```python
from build123d import *

# Parameters (mm, degrees)
SKETCH1_R           = 1.778
BOSS_EXTRUDE1_DEPTH = 6.35
SKETCH2_R           = 1.778
BOSS_EXTRUDE2_DEPTH = 6.35
SKETCH3_R           = 1.905
CUT_EXTRUDE1_DEPTH  = 103.859220114


with BuildPart() as part:
    # Sketch1 → Boss-Extrude1 (new body)
    with BuildSketch(Plane(origin=(0, 6.35, 0), x_dir=(1, 0, 0), z_dir=(0, 1, 0))):
        with BuildLine():
            Line((97.79, 4.7625), (-97.79, 4.7625))
            ThreePointArc((-97.79, 4.7625), (-102.5525, 0), (-97.79, -4.7625))
            Line((-97.79, -4.7625), (97.79, -4.7625))
            ThreePointArc((97.79, -4.7625), (102.5525, 0), (97.79, 4.7625))
        make_face()
        with Locations(Location((97.79, 0, 0), (0, 0, 90))):
            Circle(SKETCH1_R, mode=Mode.SUBTRACT)
        with Locations(Location((88.011, 0, 0), (0, 0, 90))):
            Circle(SKETCH1_R, mode=Mode.SUBTRACT)
        with Locations(Location((78.232, 0, 0), (0, 0, 90))):
            Circle(SKETCH1_R, mode=Mode.SUBTRACT)
        with Locations(Location((68.453, 0, 0), (0, 0, 90))):
            Circle(SKETCH1_R, mode=Mode.SUBTRACT)
        with Locations(Location((58.674, 0, 0), (0, 0, 90))):
            Circle(SKETCH1_R, mode=Mode.SUBTRACT)
        with Locations(Location((48.895, 0, 0), (0, 0, 90))):
            Circle(SKETCH1_R, mode=Mode.SUBTRACT)
        with Locations(Location((39.116, 0, 0), (0, 0, 90))):
            Circle(SKETCH1_R, mode=Mode.SUBTRACT)
        with Locations(Location((29.337, 0, 0), (0, 0, 90))):
            Circle(SKETCH1_R, mode=Mode.SUBTRACT)
        with Locations(Location((19.558, 0, 0), (0, 0, 90))):
            Circle(SKETCH1_R, mode=Mode.SUBTRACT)
        with Locations(Location((9.779, 0, 0), (0, 0, 90))):
            Circle(SKETCH1_R, mode=Mode.SUBTRACT)
        with Locations(Location((0, 0, 0), (0, 0, 90))):
            Circle(SKETCH1_R, mode=Mode.SUBTRACT)
        with Locations(Location((-9.779, 0, 0), (0, 0, 90))):
            Circle(SKETCH1_R, mode=Mode.SUBTRACT)
        with Locations(Location((-19.558, 0, 0), (0, 0, 90))):
            Circle(SKETCH1_R, mode=Mode.SUBTRACT)
        with Locations(Location((-29.337, 0, 0), (0, 0, 90))):
            Circle(SKETCH1_R, mode=Mode.SUBTRACT)
        with Locations(Location((-39.116, 0, 0), (0, 0, 90))):
            Circle(SKETCH1_R, mode=Mode.SUBTRACT)
        with Locations(Location((-48.895, 0, 0), (0, 0, 90))):
            Circle(SKETCH1_R, mode=Mode.SUBTRACT)
        with Locations(Location((-58.674, 0, 0), (0, 0, 90))):
            Circle(SKETCH1_R, mode=Mode.SUBTRACT)
        with Locations(Location((-68.453, 0, 0), (0, 0, 90))):
            Circle(SKETCH1_R, mode=Mode.SUBTRACT)
        with Locations(Location((-78.232, 0, 0), (0, 0, 90))):
            Circle(SKETCH1_R, mode=Mode.SUBTRACT)
        with Locations(Location((-88.011, 0, 0), (0, 0, 90))):
            Circle(SKETCH1_R, mode=Mode.SUBTRACT)
        with Locations(Location((-97.79, 0, 0), (0, 0, 90))):
            Circle(SKETCH1_R, mode=Mode.SUBTRACT)
    extrude(amount=-BOSS_EXTRUDE1_DEPTH)

    # Sketch2 → Boss-Extrude2 (add)
    with BuildSketch(Plane(origin=(0, 6.35, 0), x_dir=(1, 0, 0), z_dir=(0, 1, 0))):
        with Locations((-88.011, 0)):
            Circle(SKETCH2_R)
    extrude(amount=-BOSS_EXTRUDE2_DEPTH)

    # Sketch3 → Cut-Extrude1 (cut, through all)
    with BuildSketch(Plane(origin=(0, 6.35, 0), x_dir=(1, 0, 0), z_dir=(0, 1, 0))):
        with Locations(Location((-91.44, 0, 0), (0, 0, 270))):
            Circle(SKETCH3_R)
    extrude(amount=-CUT_EXTRUDE1_DEPTH, mode=Mode.SUBTRACT)


solid = part.part
```
Read the model definition and answer for the solid it produces. Units are mm, in the model's axes. Round coordinates to 2 decimals unless told otherwise and drop trailing zeros. Write each loop counter-clockwise with the first axis right and the second up, starting at its lowest first coordinate (ties: lowest second). Pieces come first, ordered by that corner, then holes. Notation, with made-up numbers: M 35.25,-5 L 77.25,-5 A19 ccw 77.25,27 Z; hole C -40,20.5 d6. An arc over 180 degrees is marked long. One line per item, written item: value.
Q1. Flat-ended cylindrical pins translate along their axes: pin 1 Ø2 at (x, z) = (97.79, 0) entering from -Y; pin 2 Ø3 at (x, z) = (38.5, -2) entering from -Y; pin 3 Ø1.5 at (y, z) = (1, -3) entering from +X. Find the tip coordinate at first contact, or state that the pin passes through.
Data:
pin 1: through
pin 2: y = 0
pin 3: x = 101.99
Q2. For a pull along Z with two mould halves and no side action, classify faces 1 (the cylindrical face through (102.55, 3.22, 0.1)), 2 (the flat face through (-1, 0, -2)), 3 (the cylindrical face through (47.13, 3.22, 0.23)), 4 (the flat face through (-1, 3, 4.762)) as +Z half, -Z half, draft (parallel to the pull), parting line (faces both ways), or undercut.
Data:
face 1: parting line
face 2: draft
face 3: undercut
face 4: +Z half
Q3. Straight lines are drawn through the part: line 1 (Z direction, x = 29, y = 3); line 2 (Z direction, x = 9, y = 6); line 3 (X direction, y = 3, z = -2). For each, find the intervals that lie inside material, in ascending order. Write a range as [from, to].
Data:
line 1: [-4.76, -1.75], [1.75, 4.76]
line 2: [-4.76, -1.6], [1.6, 4.76]
line 3: [-102.11, 102.11]
Q4. Find section C-C on y = 1.5. Count the separate pieces of the cut face and the enclosed holes in it, plus the area to 3 significant figures.
Data:
separate pieces: 1
enclosed holes: 21
area: 1,720 mm2
Q5. Find section B-B on x = 0. Write down the section's boundary in (y, z), plus the area to 3 significant figures.
Data:
outline: M 0,-4.76 L 6.35,-4.76 L 6.35,-1.78 L 0,-1.78 Z; M 0,1.78 L 6.35,1.78 L 6.35,4.76 L 0,4.76 Z
area: 37.9 mm2
